from build123d import *

# Parameters (mm, degrees)
SKETCH_W     = 60
SKETCH_H     = 60
SKETCH_W_2   = 54
SKETCH_H_2   = 54
PAD_DEPTH    = 921
SKETCH002_R  = 2.75
POCKET_DEPTH = 3


with BuildPart() as part:
    # Sketch → Pad (new body)
    with BuildSketch(Plane.XZ):
        Rectangle(SKETCH_W, SKETCH_H)
        Rectangle(SKETCH_W_2, SKETCH_H_2, mode=Mode.SUBTRACT)
    extrude(amount=PAD_DEPTH)

    # Sketch002 (on Face2 of Pad) → Pocket (cut)
    with BuildSketch(Plane(origin=(30, 0, 0), x_dir=(0, 0, 1), z_dir=(1, 0, 0))):
        with Locations((-20, 50)):
            Circle(SKETCH002_R)
        with Locations((20, 50)):
            Circle(SKETCH002_R)
        with Locations((-20, 10)):
            Circle(SKETCH002_R)
        with Locations((20, 10)):
            Circle(SKETCH002_R)
        with Locations((-20, 903)):
            Circle(SKETCH002_R)
        with Locations((20, 903)):
            Circle(SKETCH002_R)
        with Locations((-20, 863)):
            Circle(SKETCH002_R)
        with Locations((20, 863)):
            Circle(SKETCH002_R)
    extrude(amount=-POCKET_DEPTH, mode=Mode.SUBTRACT)


solid = part.part
Model file for the job. Use its own axes, mm. A direction names the side the tool comes from. Give positions to 0.01 mm unless a question says otherwise; leave off trailing zeros. Write each loop counter-clockwise with the first axis right and the second up, starting at its lowest first coordinate (ties: lowest second). Pieces come first, ordered by that corner, then holes. Notation, with made-up numbers: M 72,-8 L 86,-8 A33 ccw 86,31 Z; hole C 88.5,67 d5. An arc over 180 degrees is marked long. One line per item, written item: value. Start each with the question number.
Q1. Saw through at A-A, the plane x = 10. Write the cut outline in (y, z), plus the area to 3 significant figures.
Q2. Drop a flat-ended pin along its axis: pin 1 Ø3.5 at (y, z) = (-903, 20) entering from +X. Give the stop position or say it passes through.
Q3. Saw through at B-B, the plane y = -443. Write the cut outline in (x, z).
Q4. Probe probe 1 along Z at (x, y) = (28.65, -50); probe 2 along Y at (x, z) = (27.8, 20); probe 3 along X at (y, z) = (-319, 11). List the from-to ranges inside material, lowest first. Write a range as [from, to].
Q5. 3-axis set-ups, long thin cutter, end or side, ignore diameter. For faces 1 (the flat face through (-2, -921, -29)), 2 (the flat face through (27, -454, 0)): which of +Z, -Z, +X, -X, +Y, -Y reach the whole face in a straight line?
Q6. Saw through at C-C, the plane z = -2.5. Write the cut outline in (x, y), plus the area to 3 significant figures.
Q7. Two-plate mould, pull along Z, no slides. Class faces 3 (the flat face through (-27, -454, 0)), 4 (the flat face through (0, -454, -30)), 5 (the flat face through (0, -454, 27)), 6 (the flat face through (30, -454, 0)): +Z half, -Z half, draft (parallel to the pull), parting line (faces both ways), or undercut.
Output values:
1. outline: M -921,-30 L 0,-30 L 0,-27 L -921,-27 Z; M -921,27 L 0,27 L 0,30 L -921,30 Z
1. area: 5,530 mm²
2. pin 1: stops at x = -27
3. outline: M -30,-30 L 30,-30 L 30,30 L -30,30 Z; hole M -27,-27 L 27,-27 L 27,27 L -27,27 Z
4. probe 1: z = [-30, -22.75], [-17.25, 17.25], [22.75, 30]
4. probe 2: y = [-921, -905.75], [-900.25, -865.75], [-860.25, -52.75], [-47.25, -12.75], [-7.25, 0]
4. probe 3: x = [-30, -27], [27, 30]
5. face 1: +Z, -Z, +X, -X, -Y
5. face 2: +Y, -Y
6. outline: M -30,-921 L -27,-921 L -27,0 L -30,0 Z; M 27,-921 L 30,-921 L 30,0 L 27,0 Z
6. area: 5,530 mm²
7. face 3: undercut
7. face 4: -Z half
7. face 5: undercut
7. face 6: draft
